from build123d import *

# Parameters (mm, degrees)
BOSS_EXTRUDE1_DEPTH            = 30
SKETCH2_R                      = 2.6
SKETCH2_R_2                    = 1.55
BOSS_EXTRUDE3_DEPTH            = 5
CUT_EXTRUDE1_REACH             = 109.267
CUT_EXTRUDE1_DIRECTION_2_DEPTH = 108.267308909
CUT_EXTRUDE2_REACH             = 109.267
CUT_EXTRUDE2_DIRECTION_2_DEPTH = 108.267308909
FILLET1_R                      = 2
SKETCH6_R                      = 2.6
BOSS_EXTRUDE4_DEPTH            = 1


with BuildPart() as part:
    # Sketch1 → Boss-Extrude1 (new body)
    with BuildSketch(Plane(origin=(0, 0, 0), x_dir=(1, 0, 0), z_dir=(0, 1, 0))):
        Polygon((-13.5, 0), (0, 93.036251394), (13.5, 0), (14.489635693, 0.143600819), (0, 100), (-14.489635693, 0.143600819), align=None)
    extrude(amount=BOSS_EXTRUDE1_DEPTH)

    # Sketch2 → Boss-Extrude3 (add)
    # profile 1 of 8: a face of its own
    with BuildSketch(Plane(origin=(0, 0, 0), x_dir=(1, 0, 0), z_dir=(0, 1, 0))):
        with Locations((11.916582891, -0.22976131)):
            Circle(SKETCH2_R)
        with Locations(Location((11.916582891, -0.22976131, 0), (0, 0, 270))):
            Circle(SKETCH2_R_2, mode=Mode.SUBTRACT)
    # profile 2 of 8: a face of its own
    with BuildSketch(Plane(origin=(0, 0, 0), x_dir=(1, 0, 0), z_dir=(0, 1, 0))):
        with Locations((9.618969794, 15.604409779)):
            Circle(SKETCH2_R)
        with Locations(Location((9.618969794, 15.604409779, 0), (0, 0, 270))):
            Circle(SKETCH2_R_2, mode=Mode.SUBTRACT)
    # profile 3 of 8: a face of its own
    with BuildSketch(Plane(origin=(0, 0, 0), x_dir=(1, 0, 0), z_dir=(0, 1, 0))):
        with Locations((7.321356697, 31.438580867)):
            Circle(SKETCH2_R)
        with Locations(Location((7.321356697, 31.438580867, 0), (0, 0, 270))):
            Circle(SKETCH2_R_2, mode=Mode.SUBTRACT)
    # profile 4 of 8: a face of its own
    with BuildSketch(Plane(origin=(0, 0, 0), x_dir=(1, 0, 0), z_dir=(0, 1, 0))):
        with Locations((5.0237436, 47.272751956)):
            Circle(SKETCH2_R)
        with Locations(Location((5.0237436, 47.272751956, 0), (0, 0, 270))):
            Circle(SKETCH2_R_2, mode=Mode.SUBTRACT)
    # profile 5 of 8: a face of its own
    with BuildSketch(Plane(origin=(0, 0, 0), x_dir=(1, 0, 0), z_dir=(0, 1, 0))):
        with Locations((-11.916582891, -0.22976131)):
            Circle(SKETCH2_R)
        with Locations(Location((-11.916582891, -0.22976131, 0), (0, 0, 90))):
            Circle(SKETCH2_R_2, mode=Mode.SUBTRACT)
    # profile 6 of 8: a face of its own
    with BuildSketch(Plane(origin=(0, 0, 0), x_dir=(1, 0, 0), z_dir=(0, 1, 0))):
        with Locations((-9.618969794, 15.604409779)):
            Circle(SKETCH2_R)
        with Locations(Location((-9.618969794, 15.604409779, 0), (0, 0, 90))):
            Circle(SKETCH2_R_2, mode=Mode.SUBTRACT)
    # profile 7 of 8: a face of its own
    with BuildSketch(Plane(origin=(0, 0, 0), x_dir=(1, 0, 0), z_dir=(0, 1, 0))):
        with Locations((-7.321356697, 31.438580867)):
            Circle(SKETCH2_R)
        with Locations(Location((-7.321356697, 31.438580867, 0), (0, 0, 90))):
            Circle(SKETCH2_R_2, mode=Mode.SUBTRACT)
    # profile 8 of 8: a face of its own
    with BuildSketch(Plane(origin=(0, 0, 0), x_dir=(1, 0, 0), z_dir=(0, 1, 0))):
        with Locations((-5.0237436, 47.272751956)):
            Circle(SKETCH2_R)
        with Locations(Location((-5.0237436, 47.272751956, 0), (0, 0, 90))):
            Circle(SKETCH2_R_2, mode=Mode.SUBTRACT)
    boss_extrude3 = extrude(amount=BOSS_EXTRUDE3_DEPTH)

    # Cut-Extrude1: up to this face of the body (flat: up to its plane)
    cut_extrude1_end = Plane(part.part.faces().sort_by_distance((-6.677185099, 15.326206653, -47.019934992))[0])
    # Sketch4 → Cut-Extrude1 (cut, up to the picked face)
    with BuildSketch(Plane(origin=(0.278386134, 0, 1.918518691), x_dir=(0.9896356930251445, 0, -0.14360081855839762), z_dir=(0.14360081855839762, 0, 0.9896356930251445)), mode=Mode.PRIVATE) as cut_extrude1_sk1:
        Polygon((13.360081856, 5), (9.160081856, 5), (9.160081856, 1.475781549), align=None)
    cut_extrude1_tool1 = split(extrude(cut_extrude1_sk1.sketch, amount=-CUT_EXTRUDE1_REACH, mode=Mode.PRIVATE), bisect_by=cut_extrude1_end, keep=Keep.BOTH, mode=Mode.PRIVATE)
    cut_extrude1 = cut_extrude1_tool1.solids().sort_by(Axis((10.72902, 3.825261, 0.402082), (-0.14360081855839762, 0, -0.9896356930251445)))[0]
    add(cut_extrude1, mode=Mode.SUBTRACT)

    # Sketch4 → Cut-Extrude1 direction 2 (cut)
    with BuildSketch(Plane(origin=(0.278386134, 0, 1.918518691), x_dir=(0.9896356930251445, 0, -0.14360081855839762), z_dir=(0.14360081855839762, 0, 0.9896356930251445))):
        Polygon((13.360081856, 5), (9.160081856, 5), (9.160081856, 1.475781549), align=None)
    cut_extrude1_direction_2 = extrude(amount=CUT_EXTRUDE1_DIRECTION_2_DEPTH, mode=Mode.SUBTRACT)

    # Cut-Extrude2: up to this face of the body (flat: up to its plane)
    cut_extrude2_end = Plane(part.part.faces().sort_by_distance((6.677185099, 15.326206653, -47.019934992))[0])
    # Sketch5 → Cut-Extrude2 (cut, up to the picked face)
    with BuildSketch(Plane(origin=(-0.278386134, 0, 1.918518691), x_dir=(0.9896356930251446, 0, 0.14360081855839799), z_dir=(-0.14360081855839799, 0, 0.9896356930251446)), mode=Mode.PRIVATE) as cut_extrude2_sk1:
        Polygon((-9.083094078, 5), (-9.083094078, 1.411181133), (-13.360081856, 5), align=None)
    cut_extrude2_tool1 = split(extrude(cut_extrude2_sk1.sketch, amount=-CUT_EXTRUDE2_REACH, mode=Mode.PRIVATE), bisect_by=cut_extrude2_end, keep=Keep.BOTH, mode=Mode.PRIVATE)
    cut_extrude2 = cut_extrude2_tool1.solids().sort_by(Axis((-10.678227, 3.803727, 0.409453), (0.14360081855839799, 0, -0.9896356930251446)))[0]
    add(cut_extrude2, mode=Mode.SUBTRACT)

    # Sketch5 → Cut-Extrude2 direction 2 (cut)
    with BuildSketch(Plane(origin=(-0.278386134, 0, 1.918518691), x_dir=(0.9896356930251446, 0, 0.14360081855839799), z_dir=(-0.14360081855839799, 0, 0.9896356930251446))):
        Polygon((-9.083094078, 5), (-9.083094078, 1.411181133), (-13.360081856, 5), align=None)
    cut_extrude2_direction_2 = extrude(amount=CUT_EXTRUDE2_DIRECTION_2_DEPTH, mode=Mode.SUBTRACT)

    # Mirror2: Boss-Extrude3, Cut-Extrude1, Cut-Extrude1 direction 2, Cut-Extrude2, Cut-Extrude2 direction 2 across plane
    add(boss_extrude3.mirror(Plane.ZX.offset(15)))
    add(cut_extrude1.mirror(Plane.ZX.offset(15)), mode=Mode.SUBTRACT)
    add(cut_extrude1_direction_2.mirror(Plane.ZX.offset(15)), mode=Mode.SUBTRACT)
    add(cut_extrude2.mirror(Plane.ZX.offset(15)), mode=Mode.SUBTRACT)
    add(cut_extrude2_direction_2.mirror(Plane.ZX.offset(15)), mode=Mode.SUBTRACT)

    # Fillet1
    # the kernel refuses this fillet: 2 mm, written as the material it adds along each edge
    with BuildSketch(Plane(origin=(13.5, 25, 0), x_dir=(0, -1, 0), z_dir=(0.9896356930251446, 0, -0.14360081855839765))) as fillet1_piece_1_section:
        with BuildLine():
            CenterArc((FILLET1_R, -FILLET1_R), FILLET1_R, 90, 90)
            Line((0, -FILLET1_R), (0, 0))
            Line((0, 0), (FILLET1_R, 0))
        make_face()
    fillet1_piece_1 = extrude(amount=6, mode=Mode.PRIVATE)
    fillet1_piece_1 = fillet1_piece_1 & Plane(origin=(11.916582891, 24.30002226, 0.22976131), x_dir=(1, 0, 0), z_dir=(0, 1, 0)) * Cylinder(2.6, 21, mode=Mode.PRIVATE)
    add(fillet1_piece_1)
    with BuildSketch(Plane(origin=(-19.437814158, 25, -0.861604911), x_dir=(0, -1, 0), z_dir=(0.9896356930251445, 0, 0.143600818558398))) as fillet1_piece_2_section:
        with BuildLine():
            CenterArc((FILLET1_R, -FILLET1_R), FILLET1_R, 90, 90)
            Line((0, -FILLET1_R), (0, 0))
            Line((0, 0), (FILLET1_R, 0))
        make_face()
    fillet1_piece_2 = extrude(amount=6, mode=Mode.PRIVATE)
    fillet1_piece_2 = fillet1_piece_2 & Plane(origin=(-11.916582891, 24.777637105, 0.22976131), x_dir=(1, 0, 0), z_dir=(0, 1, 0)) * Cylinder(2.6, 21, mode=Mode.PRIVATE)
    add(fillet1_piece_2)
    with BuildSketch(Plane(origin=(13.5, 5, 0), x_dir=(0, 1, 0), z_dir=(0.9896356930251446, 0, -0.14360081855839765))) as fillet1_piece_3_section:
        with BuildLine():
            CenterArc((FILLET1_R, FILLET1_R), FILLET1_R, 180, 90)
            Line((0, FILLET1_R), (0, 0))
            Line((0, 0), (FILLET1_R, 0))
        make_face()
    fillet1_piece_3 = extrude(amount=6, mode=Mode.PRIVATE)
    fillet1_piece_3 = fillet1_piece_3 & Plane(origin=(11.916582891, 5.699977741, 0.22976131), x_dir=(1, 0, 0), z_dir=(0, -1, 0)) * Cylinder(2.6, 21, mode=Mode.PRIVATE)
    add(fillet1_piece_3)
    with BuildSketch(Plane(origin=(-19.437814158, 5, -0.861604911), x_dir=(-0.143600818558398, 0, 0.9896356930251445), z_dir=(0.9896356930251445, 0, 0.143600818558398))) as fillet1_piece_4_section:
        with BuildLine():
            CenterArc((FILLET1_R, -FILLET1_R), FILLET1_R, 90, 90)
            Line((0, -FILLET1_R), (0, 0))
            Line((0, 0), (FILLET1_R, 0))
        make_face()
    fillet1_piece_4 = extrude(amount=6, mode=Mode.PRIVATE)
    fillet1_piece_4 = fillet1_piece_4 & Plane(origin=(-11.916582891, 5.222362792, 0.22976131), x_dir=(1, 0, 0), z_dir=(0, -1, 0)) * Cylinder(2.6, 21, mode=Mode.PRIVATE)
    add(fillet1_piece_4)

    # Sketch6 → Boss-Extrude4 (add)
    with BuildSketch(Plane.XZ):
        with Locations((-9.618969794, -15.604409779)):
            Circle(SKETCH6_R)
        with Locations((9.618969794, -15.604409779)):
            Circle(SKETCH6_R)
        with Locations((7.321356697, -31.438580867)):
            Circle(SKETCH6_R)
        with Locations((-7.321356697, -31.438580867)):
            Circle(SKETCH6_R)
        with Locations((-5.0237436, -47.272751956)):
            Circle(SKETCH6_R)
        with Locations((5.0237436, -47.272751956)):
            Circle(SKETCH6_R)
        with Locations((11.916582891, 0.22976131)):
            Circle(SKETCH6_R)
        with Locations((-11.916582891, 0.22976131)):
            Circle(SKETCH6_R)
    extrude(amount=-BOSS_EXTRUDE4_DEPTH)


solid = part.part
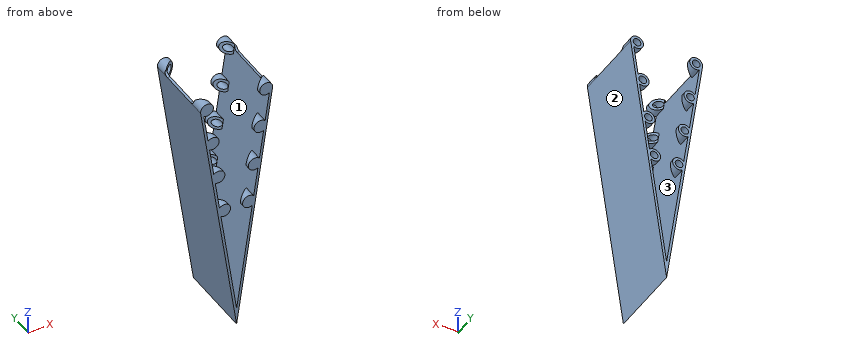
Model file for the job. Use its own axes, mm. Face numbers are marked on the shaded views. Coordinates: 2 decimals unless noted, no trailing zeros. Order: outer loops, then holes, each group sorted by start corner. A loop starts at its lowest first (then second) coordinate and runs counter-clockwise, first axis right, second up. Notation, with made-up numbers: M 56.25,45.25 L 76.25,45.25 A6 ccw 76.25,52.25 Z; hole C -29.75,19.5 d6. An arc over 180 degrees is marked long. Return JSON: item names as keys, results as strings.
1. Pull direction Z, two halves, no side cores. Call the marked faces 1, 2 and 3: +Z half, -Z half, draft (parallel to the pull), parting line (faces both ways), or undercut.
Ans:
{"face 1": "undercut", "face 2": "-Z half", "face 3": "undercut"}
2. Saw through at B-B (y = 9.5). Give the cut face in (x, z).
Ans:
{"outline": "M -14.49,-0.14 L 0,-100 L 14.49,-0.14 L 13.5,0 L 0,-93.04 L -13.5,0 Z"}
3. Flat gauge pins, fed straight in: pin 1 (2.5 mm diameter, centred on x = 9.5, z = -15.5, fed in from +Y); pin 2 (3 mm diameter, centred on y = 4.5, z = -75.5, fed in from -X). Where does each tip first touch, or does it go through?
Ans:
{"pin 1": "y = 1", "pin 2": "x = -3.77"}
4. Saw through at A-A (z = -22.5). Give the cut face in (x, y), and give its area (3 significant figures).
Ans:
{"outline": "M -11.25,0 L -10.24,0 L -10.24,30 L -11.25,30 Z; M 10.24,0 L 11.25,0 L 11.25,30 L 10.24,30 Z", "area": "60.6 mm^2"}
5. Saw through at C-C (y = 24). Give the cut face in (x, z), and give its area (3 significant figures).
Ans:
{"outline": "M -14.51,0.12 A2.6 ccw -14.49,-0.14 L 0,-100 L 14.49,-0.14 A2.6 ccw 14.51,0.12 L 13.54,0.27 L 0,-93.04 L -13.54,0.27 Z", "area": "195 mm^2"}
6. Drill centre lines: probe 1 along X at (y, z) = (21, -42); probe 2 along X at (y, z) = (12, -77.5). Where is each one in solid material? Low to high.
Ans:
{"probe 1": "-8.42 to -7.41, 7.41 to 8.42", "probe 2": "-3.26 to -2.25, 2.25 to 3.26"}
